Part model, mm, in its own coordinate system. A direction names the side the tool comes from. Round coordinates to 2 decimals unless told otherwise and drop trailing zeros. Loops run counter-clockwise (first coordinate to the right, second up) from the corner with the lowest first, then second, coordinate; pieces in that order, holes last.
1) Band-saw the part on A-A, the plane x = 32.5. Write the cut outline in (y, z), then the cut area to 3 significant figures.
2) Drop flat-ended pins along their axis: P1, Ø8, axis at x = 22.5, z = 18.5, coming from the +Y side; P2, Ø1.5, axis at x = 16.5, y = 1.5, coming from the -Z side. Give the stop position or say it passes through.
3) 3-axis set-ups, long thin cutter, end or side, ignore diameter. For faces 4 (the cylindrical face through (35.97, 5.19, -30.96)), 5 (the cylindrical face through (-34.144, 2.071, -31.548)), 6 (the flat face through (-32, 6.2, -31)): which of +Z, -Z, +X, -X, +Y, -Y reach the whole face in a straight line?
4) Band-saw the part on C-C, the plane y = 2.25. Write the cut outline in (x, z).
5) Probe line 1 (Y direction, x = -29.5, z = -23.5); line 2 (Z direction, x = 33, y = 2.75). List the from-to ranges inside material, lowest first.
6) Mould opens along Z. For faces 1 (the cylindrical face through (-34.144, 2.071, 34.952)), 2 (the flat face through (40, -2, 1)), 3 (the flat face through (-1, -2, -45)) say: +Z half, -Z half, draft (parallel to the pull), parting line (faces both ways), or undercut.
7) Band-saw the part on B-B, the plane z = 36. Write the cut outline in (x, y).
8) Band-saw the part on D-D, the plane z = -11. Write the cut outline in (x, y), then the cut area to 3 significant figures.
from build123d import *

# Parameters (mm, degrees)
SKETCH1_W           = 80
SKETCH1_H           = 90
BOSS_EXTRUDE1_DEPTH = 3.5
SKETCH2_R           = 1.95
BOSS_EXTRUDE2_DEPTH = 4.2
SKETCH3_R           = 3.5
BOSS_EXTRUDE3_DEPTH = 2


with BuildPart() as part:
    # Sketch1 → Boss-Extrude1 (new body)
    with BuildSketch(Plane(origin=(0, 0, 0), x_dir=(1, 0, 0), z_dir=(0, 1, 0))):
        Rectangle(SKETCH1_W, SKETCH1_H)
    extrude(amount=-BOSS_EXTRUDE1_DEPTH)

    # Sketch2 → Boss-Extrude2 (add)
    with BuildSketch(Plane(origin=(0, 0, 0), x_dir=(1, 0, 0), z_dir=(0, 1, 0))):
        with Locations(Location((-32.5, 30.5, 0), (0, 0, 90))):
            Circle(SKETCH2_R)
        with Locations(Location((32.5, 30.5, 0), (0, 0, 90))):
            Circle(SKETCH2_R)
        with Locations(Location((32.5, -36, 0), (0, 0, 90))):
            Circle(SKETCH2_R)
        with Locations(Location((-32.5, -36, 0), (0, 0, 90))):
            Circle(SKETCH2_R)
    extrude(amount=BOSS_EXTRUDE2_DEPTH)

    # Sketch3 → Boss-Extrude3 (add)
    with BuildSketch(Plane(origin=(0, 4.2, 0), x_dir=(1, 0, 0), z_dir=(0, 1, 0))):
        with Locations(Location((-32.5, 30.5, 0), (0, 0, 270))):
            Circle(SKETCH3_R)
        with Locations(Location((32.5, 30.5, 0), (0, 0, 270))):
            Circle(SKETCH3_R)
        with Locations(Location((-32.5, -36, 0), (0, 0, 270))):
            Circle(SKETCH3_R)
        with Locations(Location((32.5, -36, 0), (0, 0, 270))):
            Circle(SKETCH3_R)
    extrude(amount=BOSS_EXTRUDE3_DEPTH)


solid = part.part
Reported:
1. outline: (-3.5, -45) - (0, -45) - (0, -32.45) - (4.2, -32.45) - (4.2, -34) - (6.2, -34) - (6.2, -27) - (4.2, -27) - (4.2, -28.55) - (0, -28.55) - (0, 34.05) - (4.2, 34.05) - (4.2, 32.5) - (6.2, 32.5) - (6.2, 39.5) - (4.2, 39.5) - (4.2, 37.95) - (0, 37.95) - (0, 45) - (-3.5, 45) - close
1. area: 376 mm2
2. P1: stops at y = 0
2. P2: passes through
3. face 4: +Y
3. face 5: none
3. face 6: +Z, -Z, +X, -X, +Y
4. outline: circle Ø3.9 at (-32.5, -30.5); circle Ø3.9 at (-32.5, 36); circle Ø3.9 at (32.5, -30.5); circle Ø3.9 at (32.5, 36)
5. line 1: y = -3.5 to 0
5. line 2: z = -32.38 to -28.62, 34.12 to 37.88
6. face 1: undercut
6. face 2: draft
6. face 3: -Z half
7. outline: (-40, -3.5) - (40, -3.5) - (40, 0) - (34.45, 0) - (34.45, 4.2) - (36, 4.2) - (36, 6.2) - (29, 6.2) - (29, 4.2) - (30.55, 4.2) - (30.55, 0) - (-30.55, 0) - (-30.55, 4.2) - (-29, 4.2) - (-29, 6.2) - (-36, 6.2) - (-36, 4.2) - (-34.45, 4.2) - (-34.45, 0) - (-40, 0) - close
8. outline: (-40, -3.5) - (40, -3.5) - (40, 0) - (-40, 0) - close
8. area: 280 mm2
